CAD build for the part. Positions are in the model's coordinates, mm. Coordinates: 2 decimals unless noted, no trailing zeros. Loops run counter-clockwise (first coordinate to the right, second up) from the corner with the lowest first, then second, coordinate; pieces in that order, holes last.
1) Saw through at A-A, the plane z = 2.55. Write the cut outline in (x, y).
2) Saw through at B-B, the plane y = 0. Write the cut outline in (x, z), and give its area (3 significant figures).
3) Saw through at C-C, the plane x = 45. Write the cut outline in (y, z), and give its area (3 significant figures).
4) Wall check: line 1 along X through (y, z) = (1, 0.4); line 2 along Y through (x, z) = (45, 1.2); line 3 along Y through (x, z) = (70, 1.35). Give the ranges that are in metal, low to high.
5) Saw through at D-D, the plane y = 7.25. Write the cut outline in (x, z), and give its area (3 significant figures).
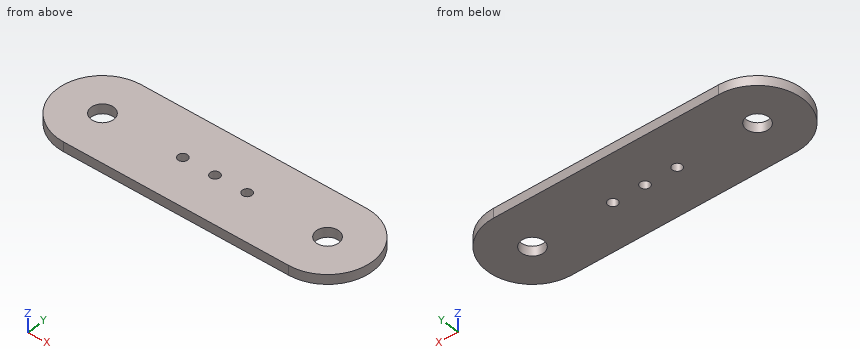
```python
from build123d import *

# Parameters (mm, degrees)
SKETCH1_R           = 1.5
SKETCH1_R_2         = 3.5
BOSS_EXTRUDE1_DEPTH = 3


with BuildPart() as part:
    # Sketch1 → Boss-Extrude1 (new body)
    with BuildSketch(Plane.XY):
        with BuildLine():
            Line((0, 14), (70, 14))
            ThreePointArc((70, 14), (84, 0), (70, -14))
            Line((70, -14), (0, -14))
            ThreePointArc((0, -14), (-14, 0), (0, 14))
        make_face()
        with Locations((25, 0)):
            Circle(SKETCH1_R, mode=Mode.SUBTRACT)
        Circle(SKETCH1_R_2, mode=Mode.SUBTRACT)
        with Locations((35, 0)):
            Circle(SKETCH1_R, mode=Mode.SUBTRACT)
        with Locations((45, 0)):
            Circle(SKETCH1_R, mode=Mode.SUBTRACT)
        with Locations((70, 0)):
            Circle(SKETCH1_R_2, mode=Mode.SUBTRACT)
    extrude(amount=BOSS_EXTRUDE1_DEPTH)


solid = part.part
```
Data:
1. outline: (0, -14) - (70, -14) arc R14 ccw to (70, 14) - (0, 14) arc R14 ccw to start; hole circle Ø7 at (0, 0); hole circle Ø3 at (25, 0); hole circle Ø3 at (35, 0); hole circle Ø3 at (45, 0); hole circle Ø7 at (70, 0)
2. outline: (-14, 0) - (-3.5, 0) - (-3.5, 3) - (-14, 3) - close; (3.5, 0) - (23.5, 0) - (23.5, 3) - (3.5, 3) - close; (26.5, 0) - (33.5, 0) - (33.5, 3) - (26.5, 3) - close; (36.5, 0) - (43.5, 0) - (43.5, 3) - (36.5, 3) - close; (46.5, 0) - (66.5, 0) - (66.5, 3) - (46.5, 3) - close; (73.5, 0) - (84, 0) - (84, 3) - (73.5, 3) - close
2. area: 225 mm2
3. outline: (-14, 0) - (-1.5, 0) - (-1.5, 3) - (-14, 3) - close; (1.5, 0) - (14, 0) - (14, 3) - (1.5, 3) - close
3. area: 75.0 mm2
4. line 1: x = -13.96 to -3.35, 3.35 to 23.88, 26.12 to 33.88, 36.12 to 43.88, 46.12 to 66.65, 73.35 to 83.96
4. line 2: y = -14 to -1.5, 1.5 to 14
4. line 3: y = -14 to -3.5, 3.5 to 14
5. outline: (-11.98, 0) - (81.98, 0) - (81.98, 3) - (-11.98, 3) - close
5. area: 282 mm2
